Autodesk Inventor part; units mm, degrees
ref_plane "YZ Plane" through (0, 0, 0) normal (1, 0, 0) x (0, 1, 0)
ref_plane "XZ Plane" through (0, 0, 0) normal (0, 1, 0) x (-1, 0, 0)
ref_plane "XY Plane" through (0, 0, 0) normal (0, 0, 1) x (1, 0, 0)
sketch "Sketch1" plane through (0, 0, 0) normal (0, 1, 0) x (-1, 0, 0)
  line L0 (27.5, 19.0625) -> (-32.5, 19.0625)
  line L1 (-32.5, 19.0625) -> (-32.5, 17.0625)
  line L2 (-32.5, 17.0625) -> (27.5, 17.0625)
  line L3 (27.5, 17.0625) -> (27.5, 19.0625)
  line L4 (27.5, 19.0625) -> (25.5, 19.0625)
  line L5 (25.5, 19.0625) -> (25.5, -20.9375)
  line L6 (25.5, -20.9375) -> (27.5, -20.9375)
  line L7 (27.5, -20.9375) -> (27.5, 19.0625)
  line L8 (-32.5, 19.0625) -> (-30.5, 19.0625)
  line L9 (-30.5, 19.0625) -> (-30.5, -20.9375)
  line L10 (-30.5, -20.9375) -> (-32.5, -20.9375)
  line L11 (-32.5, -20.9375) -> (-32.5, 19.0625)
  point P0 (0, 0)
  dimension "d0" = 2
  dimension "d1" = 0
  dimension "d2" = 2
  dimension "d3" = 2
  dimension "d4" = 60
  dimension "d5" = 40
  dimension "d6" = 40
extrude "Extrusion1" add sketch "Sketch1" along normal blind 3
fillet "Fillet1" radius 2 2 edges at (-25.5, 1.5, 17.0625) (30.5, 1.5, 17.0625)
properties part number "base extend"
CAD build for the part. Positions are in the model's coordinates, mm. A direction names the side the tool comes from. Round coordinates to 2 decimals unless told otherwise and drop trailing zeros. Order: outer loops, then holes, each group sorted by start corner. A loop starts at its lowest first (then second) coordinate and runs counter-clockwise, first axis right, second up.
Item 1: Saw through at B-B on y = 1.9. Write the cut outline in (x, z), then the cut area to 3 significant figures.
Item 2: Probe line 1 along X through (y, z) = (2.25, 15); line 2 along Z through (x, y) = (2.5, 2.55); line 3 along X through (y, z) = (1.1, 16). List the from-to ranges inside material, lowest first.
Item 3: Saw through at C-C on x = -16. Write the cut outline in (y, z).
Item 4: Saw through at A-A on z = -2. Write the cut outline in (x, y), then the cut area to 3 significant figures.
Item 5: Mould opens along X. For faces 1 (the face through (3, 1, 17.062)), 2 (the face through (-27.5, 1, -1)), 3 (the face through (3, 3, 18)) say: pulls with the +X half, pulls with the -X half, needs draft (parallel to the pull), parting line crosses it, or undercut.
Item 6: Tool access for faces 4 (the face through (31, 1, -20.938)), 5 (the face through (30.5, 1, -3)): list every direction of +Z, -Z, +X, -X, +Y, -Y with a clear straight run to the whole face (end or side of a thin tool).
Reported:
1. outline: (-27.5, -20.94) - (-25.5, -20.94) - (-25.5, 15.06) arc R2 cw to (-23.5, 17.06) - (28.5, 17.06) arc R2 cw to (30.5, 15.06) - (30.5, -20.94) - (32.5, -20.94) - (32.5, 19.06) - (-27.5, 19.06) - close
1. area: 274 mm2
2. line 1: x = -27.5 to -25.5, 30.5 to 32.5
2. line 2: z = 17.06 to 19.06
2. line 3: x = -27.5 to -25.27, 30.27 to 32.5
3. outline: (0, 17.06) - (3, 17.06) - (3, 19.06) - (0, 19.06) - close
4. outline: (-27.5, 0) - (-25.5, 0) - (-25.5, 3) - (-27.5, 3) - close; (30.5, 0) - (32.5, 0) - (32.5, 3) - (30.5, 3) - close
4. area: 12.0 mm2
5. face 1: undercut
5. face 2: pulls with the -X half
5. face 3: needs draft
6. face 4: -Z, +X, -X, +Y, -Y
6. face 5: -Z, +Y, -Y
